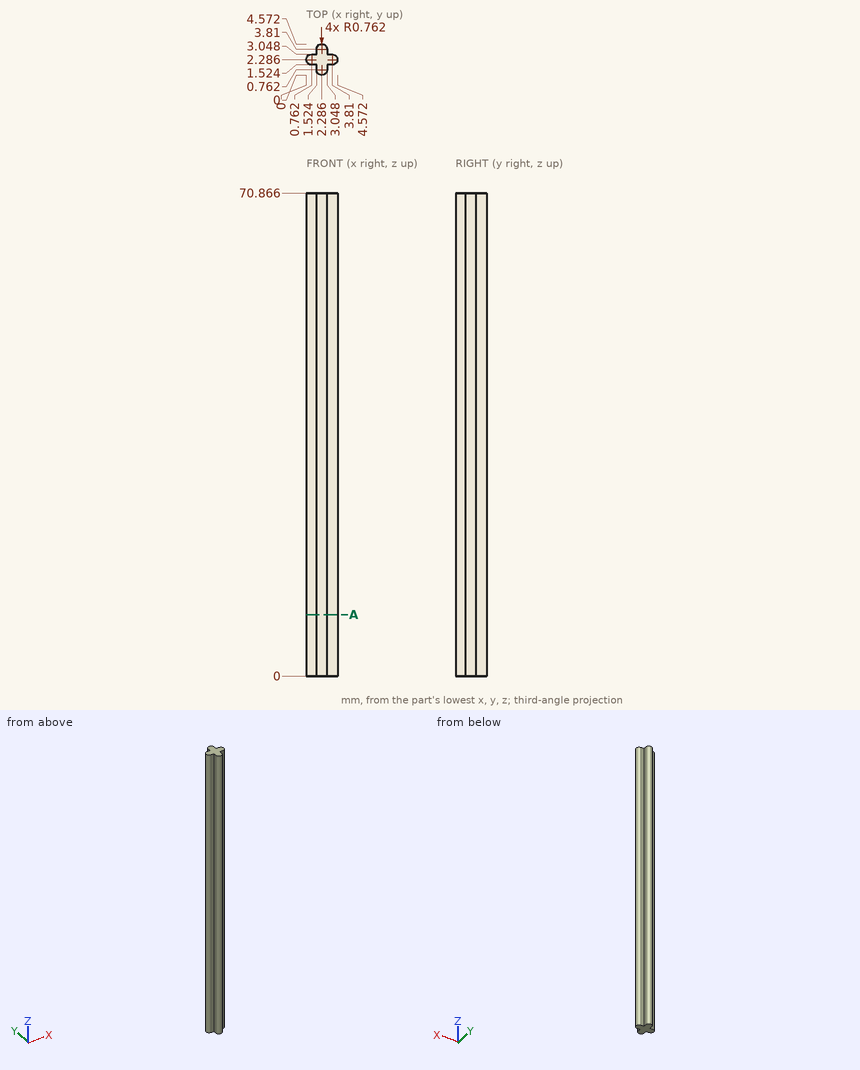
The drawing under review shows one solid part. Ordinate dimensions are in mm from its lowest x, y, z. Coordinates: 2 decimals unless noted, no trailing zeros. Order: outer loops, then holes, each group sorted by start corner. A loop starts at its lowest first (then second) coordinate and runs counter-clockwise, first axis right, second up. Notation, with made-up numbers: M 42,78.25 L 49,78.25 A24 ccw 49,108.25 Z; hole C 3.25,-6.5 d10. An arc over 180 degrees is marked long. Use a Markdown table: item, result.
(1) Wall thickness on probe 1 along X at (y, z) = (2.4, 46.5); probe 2 along X at (y, z) = (3.4, 20): over which ranges is each line inside the solid? List them lowest first.
Worked answers:
| item | result |
|---|---|
| probe 1 | x = 0.01 to 4.56 |
| probe 2 | x = 1.52 to 3.05 |
(2) For P1, Ø2, axis at y = 1.5, z = 23.5, coming from the -X side; P2, Ø1.5, axis at y = 4, z = 21.5, coming from the +X side; P3, Ø0.8, axis at x = 3.5, z = 28, coming from the -Y side, all flat-tipped, find the tip position at first contact; note any pin that passes through.
Worked answers:
| item | result |
|---|---|
| P1 | stops at x = 0 |
| P2 | stops at x = 3.05 |
| P3 | stops at y = 1.52 |
(3) Add section A-A (z = 9). Give the boundary of the cut face in (x, y), then the cut area to 3 significant figures.
Worked answers:
| item | result |
|---|---|
| outline | M 0.76,1.52 L 1.52,1.52 L 1.52,0.76 A0.76 ccw 3.05,0.76 L 3.05,1.52 L 3.81,1.52 A0.76 ccw 3.81,3.05 L 3.05,3.05 L 3.05,3.81 A0.76 ccw 1.52,3.81 L 1.52,3.05 L 0.76,3.05 A0.76 ccw Z |
| area | 10.6 mm2 |
